For this review, take the finished solid that the model builds, in its own axes (mm). Give positions to 0.01 mm unless a question says otherwise; leave off trailing zeros. Loops run counter-clockwise (first coordinate to the right, second up) from the corner with the lowest first, then second, coordinate; pieces in that order, holes last. Notation, with made-up numbers: (68, 45.25) - (125, 45.25) arc R23 cw to (125, 61.25) - close; hole circle Ø5 at (31.25, 21.25). An arc over 180 degrees is marked (long way). Answer in a Markdown table with one row per item.
```python
from build123d import *

# Parameters (mm, degrees)
SKETCH1_W           = 304.8
SKETCH1_H           = 304.8
BOSS_EXTRUDE1_DEPTH = 5.588
SKETCH2_R           = 1.6
SKETCH2_W           = 31.75
SKETCH2_H           = 25.4
SKETCH2_W_2         = 25.4
SKETCH2_H_2         = 31.75
CUT_EXTRUDE1_DEPTH  = 216.598575468


with BuildPart() as part:
    # Sketch1 → Boss-Extrude1 (new body)
    with BuildSketch(Plane(origin=(0, 0, 0), x_dir=(1, 0, 0), z_dir=(0, 1, 0))):
        Rectangle(SKETCH1_W, SKETCH1_H)
    extrude(amount=BOSS_EXTRUDE1_DEPTH)

    # Sketch2 → Cut-Extrude1 (cut, through all)
    with BuildSketch(Plane(origin=(0, 5.588, 0), x_dir=(1, 0, 0), z_dir=(0, 1, 0))):
        with Locations(Location((-107.95, 15.6, 0), (0, 0, 270))):
            Circle(SKETCH2_R)
        with Locations(Location((-69.85, 15.6, 0), (0, 0, 270))):
            Circle(SKETCH2_R)
        with Locations(Location((-107.95, -15.6, 0), (0, 0, 270))):
            Circle(SKETCH2_R)
        with Locations(Location((-69.85, -15.6, 0), (0, 0, 270))):
            Circle(SKETCH2_R)
        with Locations(Location((-15.6, -69.85, 0), (0, 0, 270))):
            Circle(SKETCH2_R)
        with Locations(Location((15.6, -69.85, 0), (0, 0, 270))):
            Circle(SKETCH2_R)
        with Locations(Location((-15.6, -107.95, 0), (0, 0, 270))):
            Circle(SKETCH2_R)
        with Locations(Location((15.6, -107.95, 0), (0, 0, 270))):
            Circle(SKETCH2_R)
        with Locations(Location((69.85, -15.6, 0), (0, 0, 270))):
            Circle(SKETCH2_R)
        with Locations(Location((69.85, 15.6, 0), (0, 0, 270))):
            Circle(SKETCH2_R)
        with Locations(Location((107.95, 15.6, 0), (0, 0, 270))):
            Circle(SKETCH2_R)
        with Locations(Location((107.95, -15.6, 0), (0, 0, 270))):
            Circle(SKETCH2_R)
        with Locations(Location((-15.6, 69.85, 0), (0, 0, 270))):
            Circle(SKETCH2_R)
        with Locations(Location((-15.6, 107.95, 0), (0, 0, 270))):
            Circle(SKETCH2_R)
        with Locations(Location((15.6, 107.95, 0), (0, 0, 270))):
            Circle(SKETCH2_R)
        with Locations(Location((15.6, 69.85, 0), (0, 0, 270))):
            Circle(SKETCH2_R)
        with Locations((-136.525, 0)):
            Rectangle(SKETCH2_W, SKETCH2_H)
        with Locations((0, 136.525)):
            Rectangle(SKETCH2_W_2, SKETCH2_H_2)
        with Locations((136.525, 0)):
            Rectangle(SKETCH2_W, SKETCH2_H)
        with Locations((0, -136.525)):
            Rectangle(SKETCH2_W_2, SKETCH2_H_2)
    extrude(amount=-CUT_EXTRUDE1_DEPTH, mode=Mode.SUBTRACT)


solid = part.part
```
1. We need section C-C, the plane x = -4. Give the boundary of the cut face in (y, z).
Values:
| item | result |
|---|---|
| outline | (0, -120.65) - (5.59, -120.65) - (5.59, 120.65) - (0, 120.65) - close |
2. We need section B-B, the plane y = 1.65. Count the separate pieces of the cut face and the enclosed holes in it, and give its area (3 significant figures).
Values:
| item | result |
|---|---|
| separate pieces | 1 |
| enclosed holes | 16 |
| area | 89,500 mm^2 |
3. Clearance check with flat-ended pins moving along their axes: pin 1 (1.7 mm diameter, centred on x = -0.5, y = 2, fed in from -Z); pin 2 (3 mm diameter, centred on x = -69.85, z = -15.6, fed in from +Y). State where each tip first meets the part, or that it passes through.
Values:
| item | result |
|---|---|
| pin 1 | stops at z = -120.65 |
| pin 2 | passes through |
4. Wall thickness on line 1 (X direction, y = 1.8, z = -15.6); line 2 (X direction, y = 1.3, z = 107.95): over which ranges is each line inside the solid? List them lowest first. Write a range as [from, to].
Values:
| item | result |
|---|---|
| line 1 | x = [-152.4, -109.55], [-106.35, -71.45], [-68.25, 68.25], [71.45, 106.35], [109.55, 152.4] |
| line 2 | x = [-152.4, -17.2], [-14, 14], [17.2, 152.4] |
5. We need section A-A, the plane x = -125. Give the boundary of the cut face in (y, z), and give its area (3 significant figures).
Values:
| item | result |
|---|---|
| outline | (0, -152.4) - (5.59, -152.4) - (5.59, -12.7) - (0, -12.7) - close; (0, 12.7) - (5.59, 12.7) - (5.59, 152.4) - (0, 152.4) - close |
| area | 1,560 mm^2 |
